Could you check a few things on this model? Use its own coordinates, in mm. Coordinates: 2 decimals unless noted, no trailing zeros. Order: outer loops, then holes, each group sorted by start corner. A loop starts at its lowest first (then second) coordinate and runs counter-clockwise, first axis right, second up. Notation, with made-up numbers: (23, 47.5) - (65, 47.5) arc R12 ccw to (65, 67.5) - close; hole circle Ø6 at (64.5, 35). An arc over 180 degrees is marked (long way). One line per item, written item: value.
from build123d import *

# Parameters (mm, degrees)
F0_R     = 11.2
F1_DEPTH = 7
F2_R     = 1.5


with BuildPart() as f1:
    # F0 (on Top) → F1 (new body)
    with BuildSketch(Plane.XY):
        with BuildLine():
            ThreePointArc((21.573992, -0.156424), (12.716124, 6.751931), (9.658758, 17.561174))
            ThreePointArc((9.658758, 17.561174), (0.778972, 39.735301), (-10.651529, 18.761837))
            ThreePointArc((-10.651529, 18.761837), (-12.205406, 7.636521), (-20.037801, -0.415857))
            ThreePointArc((-20.037801, -0.415857), (-34.801266, -19.193041), (-10.922463, -18.605414))
            ThreePointArc((-10.922463, -18.605414), (-0.510718, -14.388452), (10.379043, -17.145317))
            ThreePointArc((10.379043, -17.145317), (34.022294, -20.54226), (21.573992, -0.156424))
        make_face()
        with Locations((-23.000168, -13.279153)):
            Circle(F0_R, mode=Mode.SUBTRACT)
        with Locations((23.000168, -13.279153)):
            Circle(F0_R, mode=Mode.SUBTRACT)
        Circle(F0_R, mode=Mode.SUBTRACT)
        with Locations((0, 26.558306)):
            Circle(F0_R, mode=Mode.SUBTRACT)
    extrude(amount=F1_DEPTH)

    # F2
    f2_edges = [f1.edges().sort_by_distance(p)[0] for p in [
        (-0.510718, -14.388452, 7),
        (-34.801266, -19.193041, 7),
        (-12.205406, 7.636521, 7),
        (0.778972, 39.735301, 7),
        (12.716124, 6.751931, 7),
        (34.022294, -20.54226, 7),
    ]]
    fillet(f2_edges, radius=F2_R)


solid = f1.part
Item 1: I'm going to push flat-ended pins straight in: pin 1 Ø12 at (x, y) = (25, 10) entering from -Z; pin 2 Ø1.5 at (x, z) = (-23.5, 2) entering from +Y; pin 3 Ø4 at (x, z) = (-26.5, 2) entering from +Y. Where does each tip first touch, or does it pass through?
Conclusion:
pin 1: through
pin 2: y = -0.08
pin 3: y = -0.16
Item 2: Thinking about a two-plate mould opening in X: for faces 1 (the face through (-34.19, -12.79, 3.45)), 2 (the face through (-0.2, 11.5, 7)), 3 (the face through (33.68, -9.91, 3.45)), 4 (the face through (1.196, 39.704, 2.712)), which applies, pulls with the +X half, pulls with the -X half, needs draft (parallel to the pull), parting line crosses it, or undercut?
Conclusion:
face 1: undercut
face 2: needs draft
face 3: undercut
face 4: parting line crosses it
Item 3: I want a section at A-A on z = 2.25. Please give me the cut outline in (x, y), then the cut area to 3 significant figures.
Conclusion:
outline: (-20.04, -0.42) arc R13.2 ccw (long way) to (-10.92, -18.61) arc R18.05 cw to (10.38, -17.15) arc R13.2 ccw (long way) to (21.57, -0.16) arc R18.05 cw to (9.66, 17.56) arc R13.2 ccw (long way) to (-10.65, 18.76) arc R18.05 cw to start; hole circle Ø22.4 at (-23, -13.28); hole circle Ø22.4 at (0, 0); hole circle Ø22.4 at (0, 26.56); hole circle Ø22.4 at (23, -13.28)
area: 833 mm²
Item 4: If I drill on probe 1 along Y at (x, z) = (0, 2); probe 2 along Y at (x, z) = (-2.5, 6.75); probe 3 along X at (y, z) = (-22, 2.25), over which ranges is the centre line in solid material (lowest first)?
Conclusion:
probe 1: -14.36 to -11.2, 11.2 to 15.36, 37.76 to 39.76
probe 2: -13.95 to -10.92, 10.92 to 15.64, 37.48 to 38.84
probe 3: -32.91 to -30.03, -15.97 to -13.09, 13.09 to 15.97, 30.03 to 32.91
Item 5: I want a section at B-B on y = -22. Give the number of separate pieces and of enclosed holes in the cut face, then the cut area to 3 significant figures.
Conclusion:
separate pieces: 4
enclosed holes: 0
area: 78.0 mm²
